Job drawing, mm, ordinate dimensions from the low corner. One solid piece. A direction names the side the tool comes from. Give positions to 0.01 mm unless a question says otherwise; leave off trailing zeros. Loops run counter-clockwise (first coordinate to the right, second up) from the corner with the lowest first, then second, coordinate; pieces in that order, holes last. Notation, with made-up numbers: (-34, 1) -> (4, 1) arc R11 ccw to (4, 12) -> close; hole circle Ø9 at (-32, -15). An arc over 180 degrees is marked (long way). Answer as a JSON object with one key per item and string values. Group by question number.
Q1. Band-saw the part on A-A, the plane z = 3.04. Write the cut outline in (x, y).
Q2. Wall check: probe 1 along Z at (x, y) = (3.04, 3.8); probe 2 along Z at (x, y) = (17.5, 3.5); probe 3 along Y at (x, z) = (12.5, 18). Give the ranges that are in metal, low to high. Write a range as from..to.
Q3. Tool access for the marked faces 4, 5, 6, 7 and 8: list every direction of +Z, -Z, +X, -X, +Y, -Y with a clear straight run to the whole face (end or side of a thin tool).
Q4. Drop flat-ended pins along their axis: pin 1 (3 mm diameter, centred on y = 6.5, z = 20, fed in from +X) (3 decimals); pin 2 (2 mm diameter, centred on x = 6.5, z = 7, fed in from -Y); pin 3 (2 mm diameter, centred on x = 9.5, y = 7.5, fed in from -Z); pin 4 (2.5 mm diameter, centred on x = 17.11, z = 3.04, fed in from -Y). Give the stop position or say it passes through.
Q5. Band-saw the part on B-B, the plane x = 3.04. Write the cut outline in (y, z).
Q6. Two-plate mould, pull along Z, no slides. Class the marked faces 1, 2 and 3: pulls with the +Z half, pulls with the -Z half, needs draft (parallel to the pull), parting line crosses it, or undercut.
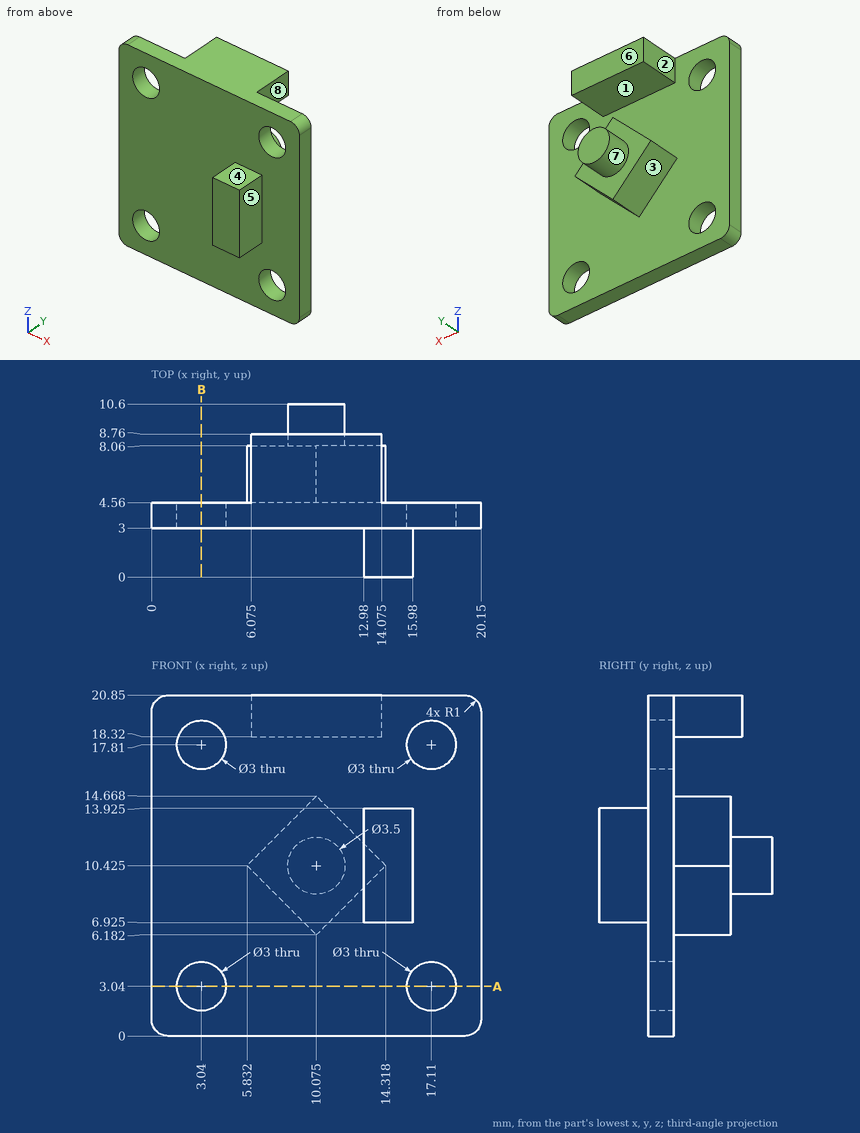
Worked answers:
{
 "1": {"outline": "(0, 3) -> (1.54, 3) -> (1.54, 4.56) -> (0, 4.56) -> close; (4.54, 3) -> (15.61, 3) -> (15.61, 4.56) -> (4.54, 4.56) -> close; (18.61, 3) -> (20.15, 3) -> (20.15, 4.56) -> (18.61, 4.56) -> close"},
 "2": {"probe 1": "0..1.54, 4.54..16.31, 19.31..20.85", "probe 2": "0..1.59, 4.49..16.36, 19.26..20.85", "probe 3": "3..4.56"},
 "3": {"face 4": "+Z, +X, -X, -Y", "face 5": "+Z, -Z, +X, -Y", "face 6": "+Z, +X, -X, +Y", "face 7": "+Y", "face 8": "+Z, +X, +Y"},
 "4": {"pin 1": "x = 14.075", "pin 2": "y = 3", "pin 3": "z = 6.18", "pin 4": "through"},
 "5": {"outline": "(3, 0) -> (4.56, 0) -> (4.56, 1.54) -> (3, 1.54) -> close; (3, 4.54) -> (4.56, 4.54) -> (4.56, 16.31) -> (3, 16.31) -> close; (3, 19.31) -> (4.56, 19.31) -> (4.56, 20.85) -> (3, 20.85) -> close"},
 "6": {"face 1": "undercut", "face 2": "needs draft", "face 3": "pulls with the -Z half"}
}
